Autodesk Inventor part; units mm, degrees
ref_plane "YZ Plane" through (0, 0, 0) normal (1, 0, 0) x (0, 1, 0)
ref_plane "XZ Plane" through (0, 0, 0) normal (0, 1, 0) x (-1, 0, 0)
ref_plane "XY Plane" through (0, 0, 0) normal (0, 0, 1) x (1, 0, 0)
sketch "Sketch1" plane through (0, 0, 0) normal (1, 0, 0) x (0, 1, 0)
  circle A0 centre (0, 0) radius 9.525
  circle A1 centre (0, 0) radius 4.7625
  dimension "d0" = 19.05
  dimension "d2" = 9.525
extrude "Extrusion1" add sketch "Sketch1" along normal mid plane 12.7
sketch "Sketch2" plane through (6.35, 0, 0) normal (1, 0, 0) x (0, 0, -1)
  circle A0 centre (0, 0) radius 12.7
  circle A1 centre (0, 0) radius 9.525 construction
  circle A2 centre (0, 0) radius 4.7625
  dimension "d6" = 3.175
extrude "Extrusion2" add sketch "Sketch2" along normal blind 1.5875
sketch "Sketch3" plane through (-6.35, 0, 0) normal (-1, 0, 0) x (0, 0, 1)
  circle A0 centre (0, 0) radius 12.7
  circle A1 centre (0, 0) radius 4.7625
extrude "Extrusion3" add sketch "Sketch3" along normal blind 1.5875
sketch "Sketch4" plane through (7.9375, 0, 0) normal (1, 0, 0) x (0, 0, -1)
  circle A0 centre (0, 0) radius 4.7625
  circle A1 centre (0, 0) radius 9.525
  dimension "d11" = 4.7625
extrude "Extrusion4" [suppressed]
properties part number "pulley XL 1.25in" material "Nylon 6/6"
The listing builds one solid part. Answer for the finished solid, in the listing's coordinates (mm). A direction names the side the tool comes from. Round coordinates to 2 decimals unless told otherwise and drop trailing zeros. Order: outer loops, then holes, each group sorted by start corner. A loop starts at its lowest first (then second) coordinate and runs counter-clockwise, first axis right, second up. Notation, with made-up numbers: (-9.5, 78.5) - (21.5, 78.5) arc R9 cw to (21.5, 94.5) - close; hole circle Ø5 at (40.5, 26). An arc over 180 degrees is marked (long way). Write item = value, one per line. Start each with the question number.
1) Straight lines are drawn through the part: L1, parallel to Z at x = 2.25, y = 0 (1 decimal); L2, parallel to Y at x = 7.2, z = 0; L3, parallel to X at y = 7.75, z = -6.75. For each, find the intervals that lie inside material, in ascending order.
2) Given pin 1 (1 mm diameter, centred on x = 5, z = -3, fed in from -Y); pin 2 (8 mm diameter, centred on x = -6, z = 7.5, fed in from -Y); pin 3 (2 mm diameter, centred on y = 3, z = 1, fed in from +X); pin 4 (1 mm diameter, centred on x = 6, z = -6, fed in from -Y), each flat-ended and moving along its own axis, determine where each tip first touches the part or whether it passes through.
3) Section D-D, the plane y = -8.75 is taken. Write down the section's boundary in (x, z), plus the area to 3 significant figures.
4) For faces 1 (the flat face through (-6.35, 9, 5)), 2 (the flat face through (-7.938, 0, 5)), determine the directions among +Z, -Z, +X, -X, +Y, -Y from which every point of the face is accessible in a straight line to the end or side of a thin tool.
5) For a pull along X with two mould halves and no side action, classify faces 3 (the flat face through (6.35, 9, -5)), 4 (the cylindrical face through (7.13, 12.4, 2.75)), 5 (the flat face through (7.938, 0, -5)) as released by +X, released by -X, zero draft, split by the parting line, or undercut.
Results list:
q1.L1 = -9.5 to -4.8, 4.8 to 9.5
q1.L2 = -12.7 to -4.76, 4.76 to 12.7
q1.L3 = -7.94 to -6.35, 6.35 to 7.94
q2.pin_1 = -9.19
q2.pin_2 = -12.2
q2.pin_3 = through
q2.pin_4 = -11.38
q3.outline = (-7.94, -9.2) - (-6.35, -9.2) - (-6.35, -3.76) - (6.35, -3.76) - (6.35, -9.2) - (7.94, -9.2) - (7.94, 9.2) - (6.35, 9.2) - (6.35, 3.76) - (-6.35, 3.76) - (-6.35, 9.2) - (-7.94, 9.2) - close
q3.area = 154 mm^2
q4.face_1 = none
q4.face_2 = +Z, -Z, -X, +Y, -Y
q5.face_3 = undercut
q5.face_4 = zero draft
q5.face_5 = released by +X
